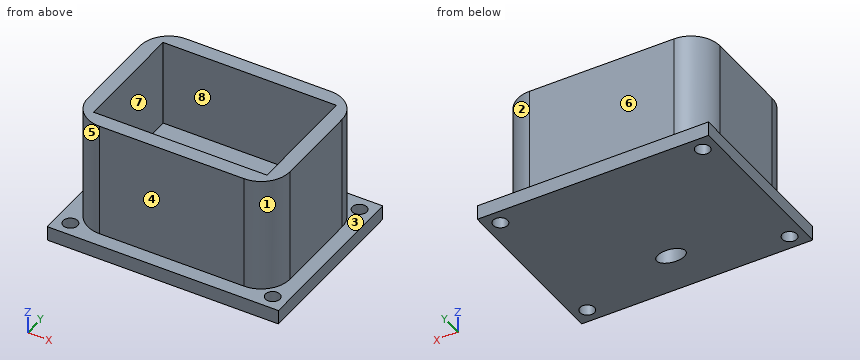
from build123d import *

# Parameters (mm, degrees)
SKETCH1_W           = 70
SKETCH1_H           = 50
BOSS_EXTRUDE1_DEPTH = 40
SKETCH2_W           = 60
SKETCH2_H           = 40
CUT_EXTRUDE1_DEPTH  = 30
BOSS_EXTRUDE2_DEPTH = 5
FILLET1_R           = 10
SKETCH5_R           = 2.5
CUT_EXTRUDE2_DEPTH  = 5
SKETCH6_RX          = 5
SKETCH6_RY          = 3
CUT_EXTRUDE3_DEPTH  = 20


with BuildPart() as part:
    # Sketch1 → Boss-Extrude1 (new body)
    with BuildSketch(Plane.XY):
        with Locations((35, 25)):
            Rectangle(SKETCH1_W, SKETCH1_H)
    extrude(amount=BOSS_EXTRUDE1_DEPTH)

    # Sketch2 → Cut-Extrude1 (cut)
    with BuildSketch(Plane.XY.offset(40)):
        with Locations((35, 25)):
            Rectangle(SKETCH2_W, SKETCH2_H)
    extrude(amount=-CUT_EXTRUDE1_DEPTH, mode=Mode.SUBTRACT)

    # Sketch4 → Boss-Extrude2 (add)
    with BuildSketch(Plane(origin=(0, 0, 0), x_dir=(-1, 0, 0), z_dir=(0, 0, -1))):
        Polygon((-75, 50), (-75, 55), (5, 55), (5, -5), (-75, -5), align=None)
    extrude(amount=BOSS_EXTRUDE2_DEPTH)

    # Fillet1
    fillet1_edges = [part.edges().sort_by_distance(p)[0] for p in [
        (0, 50, 20),
        (70, 50, 20),
        (70, 0, 20),
        (0, 0, 20),
    ]]
    fillet(fillet1_edges, radius=FILLET1_R)

    # Sketch5 → Cut-Extrude2 (cut)
    with BuildSketch(Plane.XY):
        with Locations((0, 50)):
            Circle(SKETCH5_R)
        with Locations((70, 50)):
            Circle(SKETCH5_R)
        with Locations((70, 0)):
            Circle(SKETCH5_R)
        Circle(SKETCH5_R)
    extrude(amount=-CUT_EXTRUDE2_DEPTH, mode=Mode.SUBTRACT)

    # Sketch6 → Cut-Extrude3 (cut)
    with BuildSketch(Plane.XY.offset(10)):
        with Locations(Location((35, 10), (0, 0, 180))):
            Ellipse(SKETCH6_RX, SKETCH6_RY)
    extrude(amount=-CUT_EXTRUDE3_DEPTH, mode=Mode.SUBTRACT)


solid = part.part
Part model, mm, in its own coordinate system. Face numbers are marked on the shaded views. A direction names the side the tool comes from. Coordinates: 2 decimals unless noted, no trailing zeros. Loops run counter-clockwise (first coordinate to the right, second up) from the corner with the lowest first, then second, coordinate; pieces in that order, holes last. Notation, with made-up numbers: M 34.25,-32.5 L 49.25,-32.5 A15 cw 49.25,-14.5 Z; hole C 35,28 d4. An arc over 180 degrees is marked long. Use a Markdown table: item, result. Add a question column.
Q1. Pin check, flat tips, straight feed: P1, Ø12, axis at x = 36, z = 6.5, coming from the +Y side; P2, Ø1.5, axis at y = 8, z = 4.5, coming from the -X side; P3, Ø24, axis at y = 31, z = 21.5, coming from the -X side. Stop position of each tip, or through.
Q2. Which spindle directions (+Z, -Z, +X, -X, +Y, -Y) get a long thin tool onto all of the face, cutting with end or side? Do the marked faces 1, 2, 3 and 4. Say none if no direction does.
Q3. Cut at B-B (z = 17). Write the cut outline in (x, y), and give its area (3 significant figures).
Q4. Mould opens along X. For the marked faces 5, 6, 7 and 8 say: +X half, -X half, draft (parallel to the pull), parting line (faces both ways), or undercut.
Q5. Cut at A-A (x = 69). Write the cut outline in (y, z).
Q6. Cut at C-C (y = 17). Write the cut outline in (x, z), and give its area (3 significant figures).
Q7. Cut at D-D (x = 55). Write the cut outline in (y, z), and give its area (3 significant figures).
Q8. Probe L1, parallel to Y at x = 70, z = -3.8; L2, parallel to X at y = 32, z = 19; L3, parallel to Y at x = 37.5, z = 12.5. List the from-to ranges inside material, lowest first.
Worked out:
| question | item | result |
|---|---|---|
| 1 | P1 | stops at y = 50 |
| 1 | P2 | stops at x = 0.08 |
| 1 | P3 | stops at x = 0 |
| 2 | face 1 | +Z, +X, -Y |
| 2 | face 2 | +Z, +X, +Y |
| 2 | face 3 | +Z |
| 2 | face 4 | +Z, +X, -X, -Y |
| 3 | outline | M 0,10 A10 ccw 10,0 L 60,0 A10 ccw 70,10 L 70,40 A10 ccw 60,50 L 10,50 A10 ccw 0,40 Z; hole M 5,5 L 65,5 L 65,45 L 5,45 Z |
| 3 | area | 1,010 mm2 |
| 4 | face 5 | -X half |
| 4 | face 6 | draft |
| 4 | face 7 | undercut |
| 4 | face 8 | undercut |
| 5 | outline | M -5,-5 L -2.29,-5 L -2.29,0 L -5,0 Z; M 2.29,-5 L 47.71,-5 L 47.71,0 L 44.36,0 L 44.36,40 L 5.64,40 L 5.64,0 L 2.29,0 Z; M 52.29,-5 L 55,-5 L 55,0 L 52.29,0 Z |
| 6 | outline | M -5,-5 L 75,-5 L 75,0 L 70,0 L 70,40 L 65,40 L 65,10 L 5,10 L 5,40 L 0,40 L 0,0 L -5,0 Z |
| 6 | area | 1,400 mm2 |
| 7 | outline | M -5,-5 L 55,-5 L 55,0 L 50,0 L 50,40 L 45,40 L 45,10 L 5,10 L 5,40 L 0,40 L 0,0 L -5,0 Z |
| 7 | area | 1,100 mm2 |
| 8 | L1 | y = -5 to -2.5, 2.5 to 47.5, 52.5 to 55 |
| 8 | L2 | x = 0 to 5, 65 to 70 |
| 8 | L3 | y = 0 to 5, 45 to 50 |
